Work out the finished part from the listing and answer in its coordinate system (mm). Face numbers are marked on the shaded views. A direction names the side the tool comes from. Give positions to 0.01 mm unless a question says otherwise; leave off trailing zeros. Order: outer loops, then holes, each group sorted by start corner. A loop starts at its lowest first (then second) coordinate and runs counter-clockwise, first axis right, second up. Notation, with made-up numbers: (-24, 76.5) - (-12, 76.5) arc R23 cw to (-12, 85.5) - close; hole circle Ø3 at (11, 71.25). An arc over 180 degrees is marked (long way). Write each question's results on one line, items separated by ' | '.
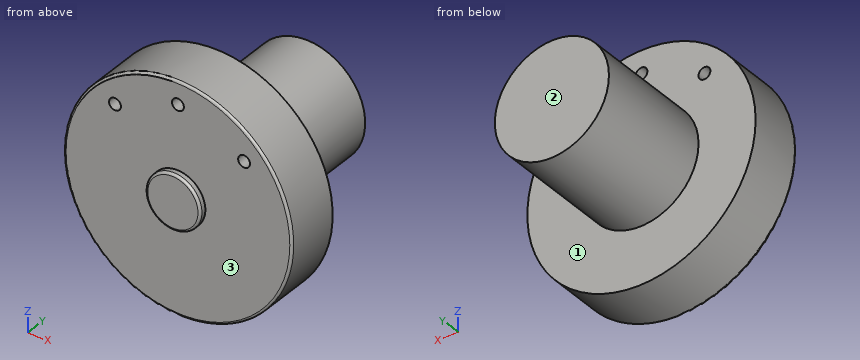
from build123d import *

# Parameters (mm, degrees)
FILLET2_R             = 0.5
F_1_0MM_DOWEL_HOLE1_D = 2.6


with BuildPart() as part:
    # Sketch1 → Revolve1 (revolve)
    with BuildSketch(Plane.XY, mode=Mode.PRIVATE) as revolve1_sk:
        Polygon((0, 0), (6, 0), (6, 1.5), (25, 1.5), (25, 13.5), (12.5, 13.5), (12.5, 40), (0, 40), align=None)
    revolve(revolve1_sk.sketch.rotate(Axis((0, 40, 0), (0, -1, 0)), 180), axis=Axis((0, 40, 0), (0, -1, 0)))

    # Fillet2
    fillet2_edges = [part.edges().sort_by_distance(p)[0] for p in [
        (25, 1.5, 0),
        (6, 0, 0),
    ]]
    fillet(fillet2_edges, radius=FILLET2_R)

    # Ø1.0mm Dowel Hole1 (through all)
    with Locations(Plane(origin=(0, 13.5, 0), x_dir=(1, 0, 0), z_dir=(0, 1, 0))):
        with Locations((14.486070668, -13.789624963), (0, -20), (-13.789624963, -14.486070668)):
            Hole(F_1_0MM_DOWEL_HOLE1_D / 2)


solid = part.part
1. Given P1, Ø3, axis at x = 14.49, z = 13.79, coming from the +Y side; P2, Ø1.5, axis at x = 18, z = -14.5, coming from the -Y side; P3, Ø10, axis at x = 1.5, y = 22, coming from the -Z side; P4, Ø2.5, axis at x = 0, z = 20, coming from the -Y side, each flat-ended and moving along its own axis, determine where each tip first touches the part or whether it passes through.
Answer list:
P1: y = 13.5 | P2: y = 1.5 | P3: z = -12.5 | P4: through
2. A cutting plane is placed at B-B, the plane z = 0. Write down the section's boundary in (x, y).
Answer list:
outline: (-25, 2) arc R0.5 ccw to (-24.5, 1.5) - (-6, 1.5) - (-6, 0.5) arc R0.5 ccw to (-5.5, 0) - (5.5, 0) arc R0.5 ccw to (6, 0.5) - (6, 1.5) - (24.5, 1.5) arc R0.5 ccw to (25, 2) - (25, 13.5) - (12.5, 13.5) - (12.5, 40) - (-12.5, 40) - (-12.5, 13.5) - (-25, 13.5) - close
3. Straight lines are drawn through the part: line 1 (X direction, y = 6, z = 14); line 2 (Y direction, x = -9.5, z = 21); line 3 (Y direction, x = 6, z = -9). For each, find the intervals that lie inside material, in ascending order. Write a range as [from, to].
Answer list:
line 1: [-20.71, -15], [-12.58, 13.2], [15.77, 20.71] | line 2: [1.5, 13.5] | line 3: [1.5, 40]
4. A cutting plane is placed at D-D, the plane y = 26.5. Write down the section's boundary in (x, z).
Answer list:
outline: circle Ø25 at (0, 0)
5. A cutting plane is placed at A-A, the plane x = 0. Write down the section's boundary in (y, z).
Answer list:
outline: (0, -5.5) arc R0.5 ccw to (0.5, -6) - (1.5, -6) - (1.5, -24.5) arc R0.5 ccw to (2, -25) - (13.5, -25) - (13.5, -12.5) - (40, -12.5) - (40, 12.5) - (13.5, 12.5) - (13.5, 18.7) - (1.5, 18.7) - (1.5, 6) - (0.5, 6) arc R0.5 ccw to (0, 5.5) - close; (1.5, 21.3) - (13.5, 21.3) - (13.5, 25) - (2, 25) arc R0.5 ccw to (1.5, 24.5) - close
6. A cutting plane is placed at C-C, the plane y = 4.5. Write down the section's boundary in (x, z).
Answer list:
outline: circle Ø50 at (0, 0); hole circle Ø2.6 at (-13.79, 14.49); hole circle Ø2.6 at (0, 20); hole circle Ø2.6 at (14.49, 13.79)
7. A tool of negligible diameter and unlimited length cuts with its end or side. For the marked faces 1, 2 and 3, from which of +Z, -Z, +X, -X, +Y, -Y can it reach the whole face along a straight path? Write none if from no direction.
Answer list:
face 1: +Y | face 2: +Z, -Z, +X, -X, +Y | face 3: -Y
